Geometry check sheet. Reference: the model listing, model coordinates, mm. Face numbers are marked on the shaded views. A direction names the side the tool comes from. Round coordinates to 2 decimals unless told otherwise and drop trailing zeros. Write each loop counter-clockwise with the first axis right and the second up, starting at its lowest first coordinate (ties: lowest second). Pieces come first, ordered by that corner, then holes. Notation, with made-up numbers: (67, -3) -> (89, -3) arc R17 ccw to (89, 13) -> close; hole circle Ø5 at (8, -31.5). An arc over 180 degrees is marked (long way). One line per question, with ' | ' between items.
```python
from build123d import *

# Parameters (mm, degrees)
SKETCH1_W           = 16.5
SKETCH1_H           = 7.8
BOSS_EXTRUDE1_DEPTH = 1
SKETCH2_W           = 18
SKETCH2_H           = 12
BOSS_EXTRUDE2_DEPTH = 3
CUT_EXTRUDE1_DEPTH  = 12
SKETCH6_R           = 0.95
CUT_EXTRUDE2_DEPTH  = 4
SKETCH8_R           = 2.5
CUT_EXTRUDE3_DEPTH  = 2.5


with BuildPart() as part:
    # Sketch1 → Boss-Extrude1 (new body)
    with BuildSketch(Plane(origin=(0, 0, 0), x_dir=(0, 0, -1), z_dir=(1, 0, 0))):
        with Locations((-8.25, 3.9)):
            Rectangle(SKETCH1_W, SKETCH1_H)
    extrude(amount=BOSS_EXTRUDE1_DEPTH)

    # Sketch2 → Boss-Extrude2 (add)
    with BuildSketch(Plane.ZY):
        with Locations((9, 3.9)):
            Rectangle(SKETCH2_W, SKETCH2_H)
    extrude(amount=BOSS_EXTRUDE2_DEPTH)

    # Sketch3 → Loft1 section 0
    with BuildSketch(Plane(origin=(0, 0, 0), x_dir=(-1, 0, 0), z_dir=(0, 0, -1))):
        Polygon((0, 7.8), (0, 9.9), (3, 9.9), (3, -2.1), (0, -2.1), (0, 0), (-1, 0), (-1, 7.8), align=None)
    # Sketch4 → Loft1 section 1
    with BuildSketch(Plane(origin=(0, 0, -21), x_dir=(-1, 0, 0), z_dir=(0, 0, -1))):
        Polygon((-11, 7.8), (-10, 7.8), (-10, 9.9), (-7, 9.9), (-7, -2.1), (-10, -2.1), (-10, 0), (-11, 0), align=None)
    loft()

    # Sketch5 → Cut-Extrude1 (cut)
    with BuildSketch(Plane(origin=(0, 9.9, 0), x_dir=(1, 0, 0), z_dir=(0, 1, 0))):
        Polygon((0, -18), (-3, -18), (-3, -16.588307156), align=None)
    extrude(amount=-CUT_EXTRUDE1_DEPTH, mode=Mode.SUBTRACT)

    # Sketch6 → Cut-Extrude2 (cut)
    with BuildSketch(Plane(origin=(1, 0, 0), x_dir=(0, 0, -1), z_dir=(1, 0, 0))):
        with Locations((-5.9, 3.9)):
            Circle(SKETCH6_R)
    extrude(amount=-CUT_EXTRUDE2_DEPTH, mode=Mode.SUBTRACT)

    # Sketch8 → Cut-Extrude3 (cut)
    with BuildSketch(Plane.ZY.offset(3)):
        with Locations((5.9, 3.9)):
            Circle(SKETCH8_R)
    extrude(amount=-CUT_EXTRUDE3_DEPTH, mode=Mode.SUBTRACT)


solid = part.part
```
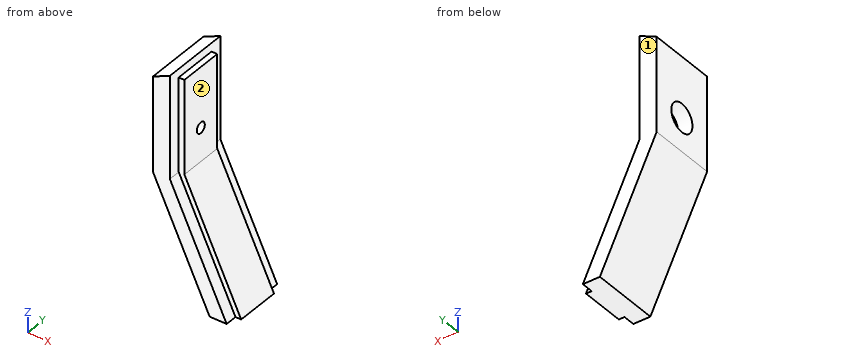
(1) Material ranges on line 1 (Y direction, x = -1.8, z = 5.9); line 2 (Y direction, x = 9.25, z = -17.5); line 3 (X direction, y = 2.75, z = 7), recorded low to high.
Resolved:
line 1: y = -2.1 to 1.4, 6.4 to 9.9 | line 2: y = 0 to 7.8 | line 3: x = -0.5 to 1
(2) Access from +Z, -Z, +X, -X, +Y, -Y to the whole of each face (thin tool, end or side, straight path). Record for the marked faces 1 and 2.
Resolved:
face 1: +Z, -Z, +X, -X, +Y | face 2: +Z, +X, +Y, -Y
(3) Sectioned sample at B-B on y = 3.9. Record the cut outline in (x, z).
Resolved:
outline: (-3, 0) -> (7, -21) -> (11, -21) -> (1, 0) -> (1, 4.95) -> (-0.5, 4.95) -> (-0.5, 3.4) -> (-3, 3.4) -> close; (-3, 8.4) -> (-0.5, 8.4) -> (-0.5, 6.85) -> (1, 6.85) -> (1, 16.5) -> (0, 16.5) -> (0, 18) -> (-3, 16.59) -> close
(4) Sectioned sample at A-A on z = 5.9. Record the cut outline in (x, y).
Resolved:
outline: (-3, -2.1) -> (0, -2.1) -> (0, 0) -> (1, 0) -> (1, 2.95) -> (-0.5, 2.95) -> (-0.5, 1.4) -> (-3, 1.4) -> close; (-3, 6.4) -> (-0.5, 6.4) -> (-0.5, 4.85) -> (1, 4.85) -> (1, 7.8) -> (0, 7.8) -> (0, 9.9) -> (-3, 9.9) -> close
(5) Sectioned sample at D-D on x = 8.5. Record the cut outline in (y, z), then the cut area to 3 significant figures.
Resolved:
outline: (-2.1, -21) -> (9.9, -21) -> (9.9, -17.85) -> (7.8, -17.85) -> (7.8, -15.75) -> (0, -15.75) -> (0, -17.85) -> (-2.1, -17.85) -> close | area: 54.2 mm2
(6) Go/stop test with flat-tipped pins: pin 1 (1 mm diameter, centred on x = 5.5, y = 3, fed in from -Z); pin 2 (6 mm diameter, centred on x = -0.5, y = 7.5, fed in from -Z); pin 3 (3 mm diameter, centred on x = 0.5, y = 1, fed in from -Z); pin 4 (4 mm diameter, centred on x = 4.5, z = 9.5, fed in from +Y). Record where each tip stops, or that it passes through.
Resolved:
pin 1: stops at z = -18.9 | pin 2: stops at z = -11.55 | pin 3: stops at z = -10.5 | pin 4: passes through
(7) Sectioned sample at C-C on x = 2.5. Record the cut outline in (y, z), then the cut area to 3 significant figures.
Resolved:
outline: (-2.1, -11.55) -> (9.9, -11.55) -> (9.9, -5.25) -> (7.8, -5.25) -> (7.8, -3.15) -> (0, -3.15) -> (0, -5.25) -> (-2.1, -5.25) -> close | area: 92.0 mm2
